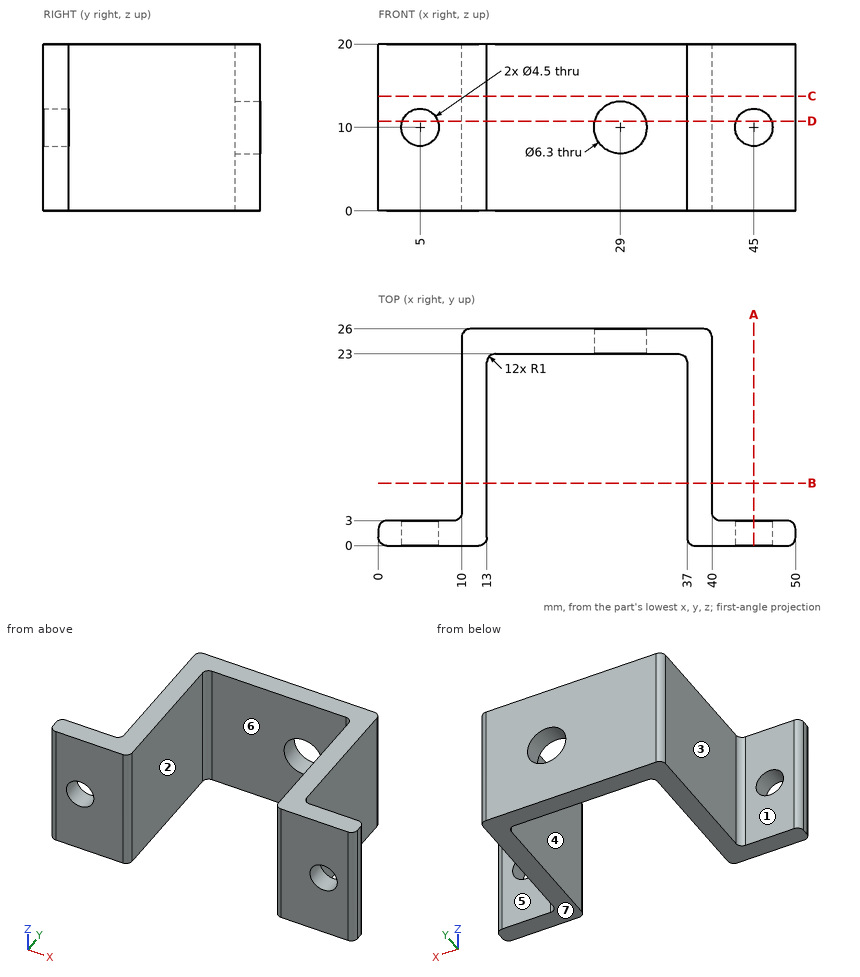
Geometry check sheet. Reference: drawing and pictorial views, mm from the part's lowest x, y, z. A direction names the side the tool comes from. Give positions to 0.01 mm unless a question says otherwise; leave off trailing zeros. Order: outer loops, then holes, each group sorted by start corner. A loop starts at its lowest first (then second) coordinate and runs counter-clockwise, first axis right, second up. Notation, with made-up numbers: M -1,67.5 L 41,67.5 A26 ccw 41,92.5 Z; hole C 37.5,43.25 d5. An arc over 180 degrees is marked long. Answer in a Markdown table with one row per item.
1) Access from +Z, -Z, +X, -X, +Y, -Y to the whole of each face (thin tool, end or side, straight path). Record for the marked faces 5, 6 and 7.
Filled sheet:
| item | result |
|---|---|
| face 5 | +Z, -Z, +X, +Y |
| face 6 | +Z, -Z, -Y |
| face 7 | -Z, +X, -X, +Y, -Y |
2) Cross-section at B-B, the plane y = 7.5. Enter the section's corners in (x, z).
Filled sheet:
| item | result |
|---|---|
| outline | M 10,0 L 13,0 L 13,20 L 10,20 Z; M 37,0 L 40,0 L 40,20 L 37,20 Z |
3) Cross-section at A-A, the plane x = 45. Enter the section's corners in (y, z), plus the area to 3 significant figures.
Filled sheet:
| item | result |
|---|---|
| outline | M 0,0 L 3,0 L 3,7.75 L 0,7.75 Z; M 0,12.25 L 3,12.25 L 3,20 L 0,20 Z |
| area | 46.5 mm2 |
4) Cross-section at C-C, the plane z = 13.75. Enter the section's corners in (x, y).
Filled sheet:
| item | result |
|---|---|
| outline | M 0,1 A1 ccw 1,0 L 12,0 A1 ccw 13,1 L 13,22 A1 cw 14,23 L 36,23 A1 cw 37,22 L 37,1 A1 ccw 38,0 L 49,0 A1 ccw 50,1 L 50,2 A1 ccw 49,3 L 41,3 A1 cw 40,4 L 40,25 A1 ccw 39,26 L 11,26 A1 ccw 10,25 L 10,4 A1 cw 9,3 L 1,3 A1 ccw 0,2 Z |
5) Gauge pin test, flat ends, axial feed: P1, Ø1, axis at y = 17.5, z = 16.5, coming from the -X side; P2, Ø8, axis at x = 29, z = 10, coming from the -Y side; P3, Ø3.5, axis at x = 45, z = 10, coming from the -Y side; P4, Ø6.5, axis at x = 6.5, z = 12, coming from the +Y side. Record the tip position at first contact, or that the pin passes through.
Filled sheet:
| item | result |
|---|---|
| P1 | stops at x = 10 |
| P2 | stops at y = 23 |
| P3 | passes through |
| P4 | stops at y = 3.34 |
6) Thickness scan on L1, parallel to Z at x = 29, y = 24.7; L2, parallel to X at y = 14, z = 8; L3, parallel to Z at x = 5, y = 0.9. Record the ranges inside material, lowest first. Write a range as [from, to].
Filled sheet:
| item | result |
|---|---|
| L1 | z = [0, 6.85], [13.15, 20] |
| L2 | x = [10, 13], [37, 40] |
| L3 | z = [0, 7.75], [12.25, 20] |
7) Release check for a two-part mould opening along X. For the marked faces 1, 2, 3 and 4 record: +X half, -X half, draft (parallel to the pull), parting line (faces both ways), or undercut.
Filled sheet:
| item | result |
|---|---|
| face 1 | draft |
| face 2 | undercut |
| face 3 | -X half |
| face 4 | undercut |
8) Cross-section at D-D, the plane z = 10.75. Count the separate pieces of the cut face and the enclosed holes in it, plus the area to 3 significant figures.
Filled sheet:
| item | result |
|---|---|
| separate pieces | 4 |
| enclosed holes | 0 |
| area | 243 mm2 |
